Read the model definition and answer for the solid it produces. Units are mm, in the model's axes. A direction names the side the tool comes from. Give positions to 0.01 mm unless a question says otherwise; leave off trailing zeros. Loops run counter-clockwise (first coordinate to the right, second up) from the corner with the lowest first, then second, coordinate; pieces in that order, holes last. Notation, with made-up numbers: (68, 42) -> (87, 42) arc R29 cw to (87, 75) -> close; hole circle Ø8 at (16.25, -15). An arc over 180 degrees is marked (long way). Write each question's results on one line, items separated by ' | '. Start each with the question number.
Item 1: Each of these flat-tipped pins is pushed along its axis until it touches: P1, Ø1.2, axis at y = 23.5, z = 0.5, coming from the +X side; P2, Ø9.5, axis at x = -43, y = -2, coming from the -Z side. Where does it stop, or does it pass through?
Item 2: Section B-B on y = -2 is taken. Write down the section's boundary in (x, z), and give its area (3 significant figures).
Item 3: Section D-D on z = 5.75 is taken. Write down the section's boundary in (x, y), and give its area (3 significant figures).
Item 4: Section A-A on x = -36 is taken. Write down the section's boundary in (y, z).
Item 5: Section C-C on y = 24 is taken. Write down the section's boundary in (x, z).
Item 6: Which of the six approach directions +Z, -Z, +X, -X, +Y, -Y give full straight-line access (tool end or side, diameter ignored) to faces 1 (the flat face through (-21.42, -15.47, -4.44)), 2 (the cylindrical face through (53.6, 22.4, -1.2)), 3 (the flat face through (1, 0, 7.5))?
Item 7: Find the intervals of material crossed by line 1 (Y direction, x = -40, z = -3.25); line 2 (Z direction, x = 52.75, y = 24); line 3 (X direction, y = 6, z = -3), in increasing order.
Item 8: Determine the mould class of faces 4 (the flat face through (46, 24, 0)), 5 (the flat face through (1, 0, -7.5)), 6 (the flat face through (-47, -4, -1.3)) for opening direction X: +X half, -X half, draft (parallel to the pull), parting line (faces both ways), or undercut.
```python
from build123d import *

# Parameters (mm, degrees)
BOSS_EXTRUDE1_DEPTH = 7.5
SKETCH2_R           = 2
CUT_EXTRUDE1_DEPTH  = 15
SKETCH3_R           = 11
CUT_EXTRUDE3_DEPTH  = 35
CUT_EXTRUDE5_DEPTH  = 6.2


with BuildPart() as part:
    # Sketch1 → Boss-Extrude1 (new, symmetric)
    with BuildSketch(Plane.XY):
        with BuildLine():
            Line((-59, 30), (59, 30))
            ThreePointArc((59, 30), (60.414213562, 29.414213562), (61, 28))
            Line((61, 28), (61, -28))
            ThreePointArc((61, -28), (60.414213562, -29.414213562), (59, -30))
            Line((59, -30), (-59, -30))
            ThreePointArc((-59, -30), (-60.414213562, -29.414213562), (-61, -28))
            Line((-61, -28), (-61, 28))
            ThreePointArc((-61, 28), (-60.414213562, 29.414213562), (-59, 30))
        make_face()
    extrude(amount=BOSS_EXTRUDE1_DEPTH, both=True)

    # Sketch2 → Cut-Extrude1 (cut)
    with BuildSketch(Plane(origin=(61, 0, 0), x_dir=(0, 0, -1), z_dir=(1, 0, 0))):
        with Locations(Location((0, 24, 0), (0, 0, 90))):
            Circle(SKETCH2_R)
        with Locations(Location((0, -24, 0), (0, 0, 270))):
            Circle(SKETCH2_R)
    extrude(amount=-CUT_EXTRUDE1_DEPTH, mode=Mode.SUBTRACT)

    # Sketch3 → Cut-Extrude3 (cut)
    with BuildSketch(Plane(origin=(0, 0, -7.5), x_dir=(-1, 0, 0), z_dir=(0, 0, -1))):
        with Locations((36, -0.850791996)):
            Circle(SKETCH3_R)
    extrude(amount=-CUT_EXTRUDE3_DEPTH, mode=Mode.SUBTRACT)

    # Sketch6 → Cut-Extrude5 (cut)
    with BuildSketch(Plane(origin=(0, 0, -7.5), x_dir=(-1, 0, 0), z_dir=(0, 0, -1))):
        Polygon((49.1, 15.249208004), (52.1, 12.249208004), (52.1, -13.950791996), (49.1, -16.950791996), (22.9, -16.950791996), (19.9, -13.950791996), (19.9, 12.249208004), (22.9, 15.249208004), align=None)
    extrude(amount=-CUT_EXTRUDE5_DEPTH, mode=Mode.SUBTRACT)


solid = part.part
```
Findings:
1) P1: x = 46 | P2: z = -1.3
2) outline: (-61, -7.5) -> (-52.1, -7.5) -> (-52.1, -1.3) -> (-46.94, -1.3) -> (-46.94, 7.5) -> (-61, 7.5) -> close; (-25.06, -1.3) -> (-19.9, -1.3) -> (-19.9, -7.5) -> (61, -7.5) -> (61, 7.5) -> (-25.06, 7.5) -> close | area: 1,440 mm2
3) outline: (-61, -28) arc R2 ccw to (-59, -30) -> (59, -30) arc R2 ccw to (61, -28) -> (61, 28) arc R2 ccw to (59, 30) -> (-59, 30) arc R2 ccw to (-61, 28) -> close; hole circle Ø22 at (-36, -0.85) | area: 6,940 mm2
4) outline: (-30, -7.5) -> (-16.95, -7.5) -> (-16.95, -1.3) -> (-11.85, -1.3) -> (-11.85, 7.5) -> (-30, 7.5) -> close; (10.15, -1.3) -> (15.25, -1.3) -> (15.25, -7.5) -> (30, -7.5) -> (30, 7.5) -> (10.15, 7.5) -> close
5) outline: (-61, -7.5) -> (61, -7.5) -> (61, -2) -> (46, -2) -> (46, 2) -> (61, 2) -> (61, 7.5) -> (-61, 7.5) -> close
6) face 1: -Z | face 2: +X | face 3: +Z, +X, -X, +Y, -Y
7) line 1: -30 to -16.95, 15.25 to 30 | line 2: -7.5 to -2, 2 to 7.5 | line 3: -61 to -52.1, -19.9 to 61
8) face 4: +X half | face 5: draft | face 6: undercut
